Model file for the job. Use its own axes, mm. Face numbers are marked on the shaded views. A direction names the side the tool comes from. Give positions to 0.01 mm unless a question says otherwise; leave off trailing zeros. Loops run counter-clockwise (first coordinate to the right, second up) from the corner with the lowest first, then second, coordinate; pieces in that order, holes last. Notation, with made-up numbers: M 64.5,-39.75 L 86.5,-39.75 A16 ccw 86.5,-19.75 Z; hole C 6,36 d9. An arc over 180 degrees is marked long. Answer in a Markdown table with one row per item.
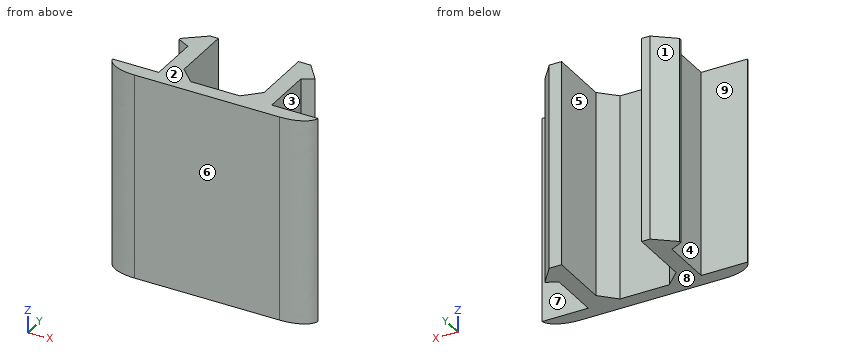
```python
from build123d import *
from OCP.BRepFilletAPI import BRepFilletAPI_MakeChamfer

# Parameters (mm, degrees)
BOSS_EXTRUDE1_DEPTH = 10
FILLET1_START       = -1
FILLET1_DEPTH       = 12
FILLET2_SIZE        = 1
FILLET2_SIZE2       = 0.8
FILLET3_SIZE        = 0.3
FILLET3_SIZE_2      = 0.6
FILLET4_SIZE        = 0.75


with BuildPart() as part:
    # Sketch1 → Boss-Extrude1 (new body)
    with BuildSketch(Plane.XY):
        Polygon((0, 0), (0, 0.7), (2.25, 0.7), (2.25, 3.2), (1.65, 3.2), (1.65, 4.4), (3.05, 4.4), (3.05, 0.7), (6.95, 0.7), (6.95, 4.4), (8.35, 4.4), (8.35, 3.2), (7.75, 3.2), (7.75, 0.7), (10, 0.7), (10, 0), align=None)
    extrude(amount=BOSS_EXTRUDE1_DEPTH)

    # Fillet1: read off the stored shape, not the designer's step
    # Fillet1 outline → Fillet1 (cut)
    with BuildSketch(Plane.XY.offset(FILLET1_START)):
        with BuildLine():
            Line((0, 0), (1.469693846, 0))
            add(Edge.make_bspline(
                [(1.469693846, 0), (0.142886902, 0), (0, 0.7)],
                knots=[0, 0, 0, 1, 1, 1], degree=2, weights=[1, 0.774596669, 1]))
            Line((0, 0.7), (0, 0))
        make_face()
        with BuildLine():
            add(Edge.make_bspline(
                [(10, 0.7), (9.857113098, 0), (8.530306154, 0)],
                knots=[0, 0, 0, 1, 1, 1], degree=2, weights=[1, 0.774596669, 1]))
            Line((8.530306154, 0), (10, 0))
            Line((10, 0), (10, 0.7))
        make_face()
    extrude(amount=FILLET1_DEPTH, mode=Mode.SUBTRACT)

    # Fillet2: one chamfer whose edges measure the first distance from different faces: ONE call of the kernel's chamfer builder (chamfer() names one face for all edges)
    fillet2_edges_1 = [part.edges().sort_by_distance(p)[0] for p in [
        (1.65, 4.4, 5),
    ]]
    fillet2_side_1 = [part.faces().sort_by_distance(p)[0] for p in [
        (2.35, 4.4, 5),
    ]]
    fillet2_edges_2 = [part.edges().sort_by_distance(p)[0] for p in [
        (8.35, 4.4, 5),
    ]]
    fillet2_side_2 = [part.faces().sort_by_distance(p)[0] for p in [
        (8.35, 3.8, 5),
    ]]
    fillet2 = BRepFilletAPI_MakeChamfer(part.part.solid().wrapped)
    for e in fillet2_edges_1:
        fillet2.Add(FILLET2_SIZE, FILLET2_SIZE2, e.wrapped, fillet2_side_1[0].wrapped)  # the first distance lies on this face
    for e in fillet2_edges_2:
        fillet2.Add(FILLET2_SIZE, FILLET2_SIZE2, e.wrapped, fillet2_side_2[0].wrapped)  # the first distance lies on this face
    add(Compound.cast(fillet2.Shape()), mode=Mode.REPLACE)

    # Fillet3
    # the kernel refuses this chamfer: 0.6, 0.3 mm, written as the material it takes off along each edge
    with BuildSketch(Plane(origin=(1.65, 3.2, -1.553897324), x_dir=(0, 1, 0), z_dir=(0, 0, 1))) as fillet3_piece_1_section:
        Polygon((FILLET3_SIZE, 0), (0, -FILLET3_SIZE_2), (0, 0), align=None)
    fillet3_piece_1 = extrude(amount=13.107794649, mode=Mode.PRIVATE)
    fillet3_piece_1 = split(fillet3_piece_1, bisect_by=Plane(origin=(2.25, 3.2, -1.553897324), z_dir=(-1, 0, 0)), keep=Keep.TOP, mode=Mode.PRIVATE)
    add(fillet3_piece_1, mode=Mode.SUBTRACT)
    with BuildSketch(Plane(origin=(8.35, 3.2, -1.553897324), x_dir=(0, 1, 0), z_dir=(0, 0, 1))) as fillet3_piece_2_section:
        Polygon((FILLET3_SIZE, 0), (0, FILLET3_SIZE_2), (0, 0), align=None)
    fillet3_piece_2 = extrude(amount=13.107794649, mode=Mode.PRIVATE)
    fillet3_piece_2 = split(fillet3_piece_2, bisect_by=Plane(origin=(7.75, 3.2, -1.553897324), z_dir=(1, 0, 0)), keep=Keep.TOP, mode=Mode.PRIVATE)
    add(fillet3_piece_2, mode=Mode.SUBTRACT)

    # Fillet4
    fillet4_edges = [part.edges().sort_by_distance(p)[0] for p in [
        (3.05, 0.7, 5),
        (6.95, 0.7, 5),
    ]]
    chamfer(fillet4_edges, length=FILLET4_SIZE)


solid = part.part
```
Q1. Saw through at A-A (y = 0.9). Give the cut face in (x, z).
Reported:
| item | result |
|---|---|
| outline | M 2.25,0 L 3.6,0 L 3.6,10 L 2.25,10 Z; M 6.4,0 L 7.75,0 L 7.75,10 L 6.4,10 Z |
Q2. Mould opens along Y. For the marked faces 6, 7, 8 and 9 say: released by +Y, released by -Y, zero draft, split by the parting line, or undercut.
Reported:
| item | result |
|---|---|
| face 6 | released by -Y |
| face 7 | undercut |
| face 8 | zero draft |
| face 9 | undercut |
Q3. 3-axis set-ups, long thin cutter, end or side, ignore diameter. For the marked faces 1, 2, 3, 4 and 5: which of +Z, -Z, +X, -X, +Y, -Y reach the whole face in a straight line?
Reported:
| item | result |
|---|---|
| face 1 | +Z, -Z, -X, +Y |
| face 2 | +Z, +X, -X, +Y, -Y |
| face 3 | +Z, -Z, +X |
| face 4 | +Z, -Z, -X |
| face 5 | +Z, -Z, +Y |
Q4. Saw through at B-B (x = 2). Give the cut face in (y, z) (3 decimals).
Reported:
| item | result |
|---|---|
| outline | M 0,0 L 0.7,0 L 0.7,10 L 0,10 Z; M 3.325,0 L 3.88,0 L 3.88,10 L 3.325,10 Z |
Q5. Drop flat-ended pins along their axis: pin 1 (1.2 mm diameter, centred on x = 5, z = 6, fed in from +Y); pin 2 (0.8 mm diameter, centred on y = 2, z = 3, fed in from -X); pin 3 (1.5 mm diameter, centred on y = 2.5, z = 7, fed in from +X). Give the stop position or say it passes through.
Reported:
| item | result |
|---|---|
| pin 1 | y = 0.7 |
| pin 2 | x = 2.25 |
| pin 3 | x = 7.85 |
Q6. Saw through at C-C (x = 4.5). Give the cut face in (y, z).
Reported:
| item | result |
|---|---|
| outline | M 0,0 L 0.7,0 L 0.7,10 L 0,10 Z |
Q7. Probe probe 1 along X at (y, z) = (2.2, 7); probe 2 along Y at (x, z) = (6, 1.5); probe 3 along X at (y, z) = (1.4, 1.25). List the from-to ranges inside material, lowest first.
Reported:
| item | result |
|---|---|
| probe 1 | 2.25 to 3.05, 6.95 to 7.75 |
| probe 2 | 0 to 0.7 |
| probe 3 | 2.25 to 3.1, 6.9 to 7.75 |
